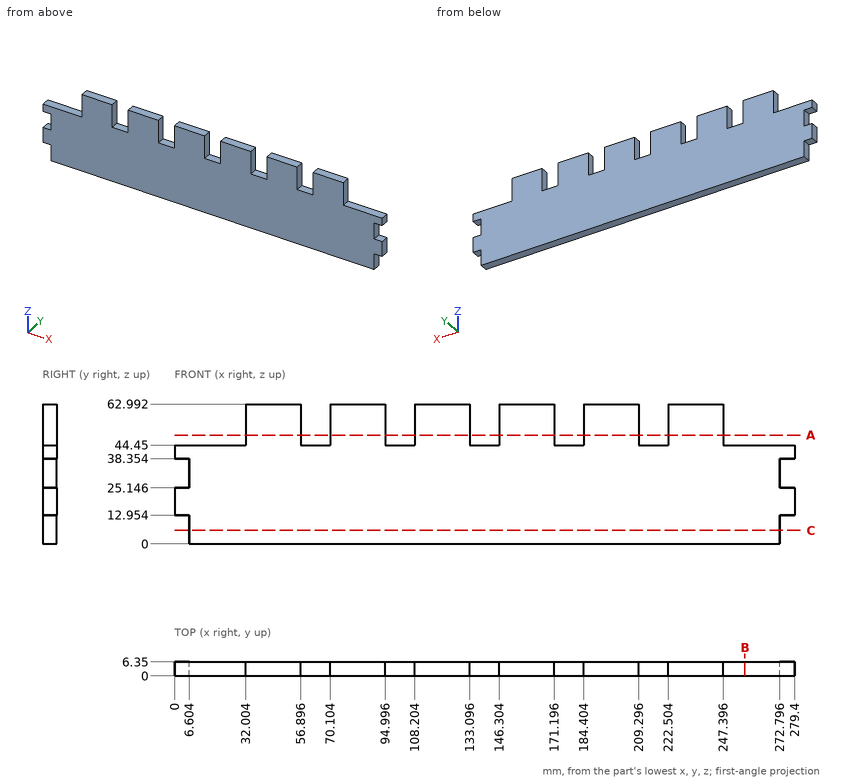
Source: three-view drawing plus pictorial views. Frame: mm from the lowest corner of the part. Round coordinates to 2 decimals unless told otherwise and drop trailing zeros. Order: outer loops, then holes, each group sorted by start corner. A loop starts at its lowest first (then second) coordinate and runs counter-clockwise, first axis right, second up. Notation, with made-up numbers: (-6, 83) -> (11, 83) arc R37 cw to (11, 119) -> close; hole circle Ø9 at (-33, -37). An arc over 180 degrees is marked (long way). Use one line per item in the form item = value.
(1) Section A-A on z = 49. Return loops of the section in (x, y).
Results list:
outline = (32, 0) -> (56.9, 0) -> (56.9, 6.35) -> (32, 6.35) -> close; (70.1, 0) -> (95, 0) -> (95, 6.35) -> (70.1, 6.35) -> close; (108.2, 0) -> (133.1, 0) -> (133.1, 6.35) -> (108.2, 6.35) -> close; (146.3, 0) -> (171.2, 0) -> (171.2, 6.35) -> (146.3, 6.35) -> close; (184.4, 0) -> (209.3, 0) -> (209.3, 6.35) -> (184.4, 6.35) -> close; (222.5, 0) -> (247.4, 0) -> (247.4, 6.35) -> (222.5, 6.35) -> close
(2) Section B-B on x = 257. Return loops of the section in (y, z).
Results list:
outline = (0, 0) -> (6.35, 0) -> (6.35, 44.45) -> (0, 44.45) -> close
(3) Section C-C on z = 6. Return loops of the section in (x, y).
Results list:
outline = (6.6, 0) -> (272.8, 0) -> (272.8, 6.35) -> (6.6, 6.35) -> close
(4) First-contact query: pin 1 Ø1.9 at (x, y) = (256, 4.5) entering from +Z; pin 2 Ø1.9 at (y, z) = (2.5, 55.5) entering from +X; pin 3 Ø1.9 at (x, y) = (275.5, 2.5) entering from +Z; pin 4 Ø5 at (x, z) = (59.5, 14) entering from -Y. Flat tips, straight axial feed; report the tip coordinate or a pass-through.
Results list:
pin_1 = 44.45
pin_2 = 247.4
pin_3 = 44.45
pin_4 = 0
(5) Ray query, probe 1 along X at (y, z) = (0.5, 58); probe 2 along Z at (x, y) = (174, 1.5); probe 3 along X at (y, z) = (2.75, 27.5). Return the intervals inside material, ascending. Write a range as [from, to].
Results list:
probe_1 = [32, 56.9], [70.1, 95], [108.2, 133.1], [146.3, 171.2], [184.4, 209.3], [222.5, 247.4]
probe_2 = [0, 44.45]
probe_3 = [6.6, 272.8]
